The listing builds one solid part. Answer for the finished solid, in the listing's coordinates (mm). Face numbers are marked on the shaded views. A direction names the side the tool comes from. Round coordinates to 2 decimals unless told otherwise and drop trailing zeros. Loops run counter-clockwise (first coordinate to the right, second up) from the corner with the lowest first, then second, coordinate; pieces in that order, holes last. Notation, with made-up numbers: (63, 53.5) -> (118, 53.5) arc R34 cw to (118, 83.5) -> close; hole circle Ø8 at (30, 1). An arc over 180 degrees is marked (long way). Use a Markdown table: item, result. Add a question column.
Q1. Section C-C on z = 14.5 is taken. Give the vertices of the cut face in (x, y), then the cut area to 3 significant figures.
Q2. Section B-B on x = 22.5 is taken. Give the vertices of the cut face in (y, z), then the cut area to 3 significant figures.
Q3. For a pull along Y with two mould halves and no side action, classify the marked faces 3, 4 and 5 as released by +Y, released by -Y, zero draft, split by the parting line, or undercut.
Q4. Section A-A on z = 28.5 is taken. Give the vertices of the cut face in (x, y), then the cut area to 3 significant figures.
Q5. Which of the six approach directions +Z, -Z, +X, -X, +Y, -Y give full straight-line access (tool end or side, diameter ignored) to the marked faces 1 and 2?
Q6. Consider line 1 (Y direction, x = 22.5, z = 29); line 2 (Y direction, x = 24, z = 7); line 3 (X direction, y = 92, z = 32). Determine where each line is inside the solid, lowest interval first.
from build123d import *

# Parameters (mm, degrees)
SKETCH1_W           = 45
SKETCH1_H           = 105
BOSS_EXTRUDE1_DEPTH = 40
SKETCH2_R           = 5.25
CUT_EXTRUDE1_DEPTH  = 17.5
SKETCH7_R           = 2.5
SKETCH6_R           = 5.25
LPATTERN1_COUNT     = 4
LPATTERN1_PITCH     = 25
FILLET1_R           = 5


with BuildPart() as part:
    # Sketch1 → Boss-Extrude1 (new body)
    with BuildSketch(Plane.XY):
        with Locations((22.5, 52.5)):
            Rectangle(SKETCH1_W, SKETCH1_H)
    extrude(amount=BOSS_EXTRUDE1_DEPTH)

    # Sketch2 → Cut-Extrude1 (cut)
    with BuildSketch(Plane.XY.offset(40)):
        with Locations((22.5, 90)):
            Circle(SKETCH2_R)
    cut_extrude1 = extrude(amount=-CUT_EXTRUDE1_DEPTH, mode=Mode.SUBTRACT)

    # Sketch7 → Cut-Loft1 section 0
    with BuildSketch(Plane.XY.offset(7.5)):
        with Locations((22.5, 90)):
            Circle(SKETCH7_R)
    # Sketch6 → Cut-Loft1 section 1
    with BuildSketch(Plane.XY.offset(22.5)):
        with Locations((22.5, 90)):
            Circle(SKETCH6_R)
    cut_loft1 = loft(mode=Mode.SUBTRACT)

    # Sketch8 → Cut-Revolve1 (revolve, cut)
    with BuildSketch(Plane.XY.offset(7.5)):
        with BuildLine():
            Line((22.5, 92.5), (22.5, 87.5))
            ThreePointArc((22.5, 87.5), (20, 90), (22.5, 92.5))
        make_face()
    cut_revolve1 = revolve(axis=Axis((22.5, 105, 7.5), (0, 1, 0)), mode=Mode.SUBTRACT)

    # LPattern1: Cut-Extrude1, Cut-Loft1, Cut-Revolve1 ×4
    with Locations(*[(0, -i * LPATTERN1_PITCH, 0) for i in range(1, LPATTERN1_COUNT)]):
        add(cut_extrude1, mode=Mode.SUBTRACT)
        add(cut_loft1, mode=Mode.SUBTRACT)
        add(cut_revolve1, mode=Mode.SUBTRACT)

    # Fillet1
    fillet1_edges = [part.edges().sort_by_distance(p)[0] for p in [
        (0, 105, 20),
        (45, 105, 20),
        (45, 0, 20),
        (0, 0, 20),
    ]]
    fillet(fillet1_edges, radius=FILLET1_R)


solid = part.part
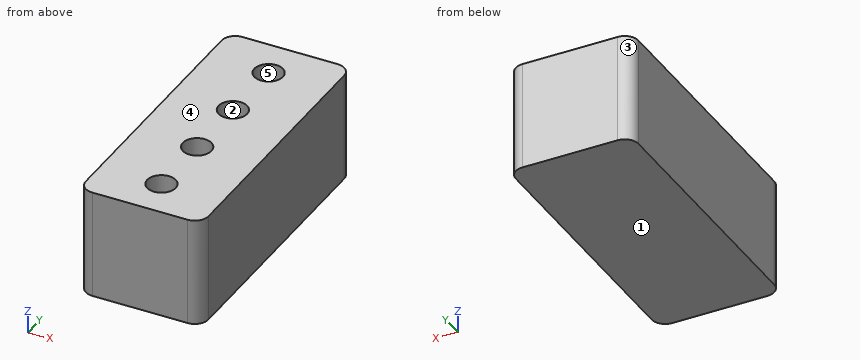
Checked values:
| question | item | result |
|---|---|---|
| 1 | outline | (0, 5) arc R5 ccw to (5, 0) -> (40, 0) arc R5 ccw to (45, 5) -> (45, 100) arc R5 ccw to (40, 105) -> (5, 105) arc R5 ccw to (0, 100) -> close; hole circle Ø7.57 at (22.5, 15); hole circle Ø7.57 at (22.5, 40); hole circle Ø7.57 at (22.5, 65); hole circle Ø7.57 at (22.5, 90) |
| 1 | area | 4,520 mm2 |
| 2 | outline | (0, 0) -> (105, 0) -> (105, 40) -> (95.25, 40) -> (95.25, 22.5) -> (92.5, 7.5) arc R2.5 cw to (87.5, 7.5) -> (84.75, 22.5) -> (84.75, 40) -> (70.25, 40) -> (70.25, 22.5) -> (67.5, 7.5) arc R2.5 cw to (62.5, 7.5) -> (59.75, 22.5) -> (59.75, 40) -> (45.25, 40) -> (45.25, 22.5) -> (42.5, 7.5) arc R2.5 cw to (37.5, 7.5) -> (34.75, 22.5) -> (34.75, 40) -> (20.25, 40) -> (20.25, 22.5) -> (17.5, 7.5) arc R2.5 cw to (12.5, 7.5) -> (9.75, 22.5) -> (9.75, 40) -> (0, 40) -> close |
| 2 | area | 2,960 mm2 |
| 3 | face 3 | released by +Y |
| 3 | face 4 | zero draft |
| 3 | face 5 | undercut |
| 4 | outline | (0, 5) arc R5 ccw to (5, 0) -> (40, 0) arc R5 ccw to (45, 5) -> (45, 100) arc R5 ccw to (40, 105) -> (5, 105) arc R5 ccw to (0, 100) -> close; hole circle Ø10.5 at (22.5, 15); hole circle Ø10.5 at (22.5, 40); hole circle Ø10.5 at (22.5, 65); hole circle Ø10.5 at (22.5, 90) |
| 4 | area | 4,360 mm2 |
| 5 | face 1 | -Z, +X, -X, +Y, -Y |
| 5 | face 2 | +Z |
| 6 | line 1 | y = 0 to 9.75, 20.25 to 34.75, 45.25 to 59.75, 70.25 to 84.75, 95.25 to 105 |
| 6 | line 2 | y = 0 to 13.06, 16.94 to 38.06, 41.94 to 63.06, 66.94 to 88.06, 91.94 to 105 |
| 6 | line 3 | x = 0 to 17.65, 27.35 to 45 |
